CAD build for the part. Positions are in the model's coordinates, mm. A direction names the side the tool comes from. Coordinates: 2 decimals unless noted, no trailing zeros. Write each loop counter-clockwise with the first axis right and the second up, starting at its lowest first coordinate (ties: lowest second). Pieces come first, ordered by that corner, then holes. Notation, with made-up numbers: (42.5, 18.25) -> (96.5, 18.25) arc R10 cw to (96.5, 37.25) -> close; hole circle Ø6 at (21, 65.25). An arc over 180 degrees is marked (long way). Answer as CSV lines item,"result".
```python
from build123d import *

# Parameters (mm, degrees)
SKETCH_1_R          = 30
EXTRUDE_1_DEPTH     = 35
SKETCH_2_R          = 1.65
CUT_EXTRUDE_1_DEPTH = 56
SKETCH_4_R          = 20
CUT_EXTRUDE_3_DEPTH = 10
SKETCH_5_R          = 4
CUT_EXTRUDE_4_DEPTH = 50.244289009
SKETCH_6_R          = 2.15
SKETCH_6_R_2        = 1.55
CUT_EXTRUDE_5_DEPTH = 50.244289009


with BuildPart() as part:
    # 草图1 → 凸台-拉伸1 (new body)
    with BuildSketch(Plane(origin=(0, 0, 0), x_dir=(1, 0, 0), z_dir=(0, 1, 0))):
        with Locations(Location((0, 0, 0), (0, 0, 270))):
            Circle(SKETCH_1_R)
    extrude(amount=EXTRUDE_1_DEPTH)

    # 草图2 → 切除-拉伸1 (cut, through all)
    with BuildSketch(Plane.XZ):
        with Locations(Location((-26.25, 0, 0), (0, 0, 270))):
            Circle(SKETCH_2_R)
        with Locations(Location((-20.108666632, 16.873174754, 0), (0, 0, 270))):
            Circle(SKETCH_2_R)
        with Locations(Location((-4.558264664, 25.851203517, 0), (0, 0, 270))):
            Circle(SKETCH_2_R)
        with Locations(Location((13.125, 22.733166849, 0), (0, 0, 270))):
            Circle(SKETCH_2_R)
        with Locations(Location((24.666931296, 8.978028762, 0), (0, 0, 270))):
            Circle(SKETCH_2_R)
        with Locations(Location((24.666931296, -8.978028762, 0), (0, 0, 270))):
            Circle(SKETCH_2_R)
        with Locations(Location((13.125, -22.733166849, 0), (0, 0, 270))):
            Circle(SKETCH_2_R)
        with Locations(Location((-4.558264664, -25.851203517, 0), (0, 0, 270))):
            Circle(SKETCH_2_R)
        with Locations(Location((-20.108666632, -16.873174754, 0), (0, 0, 270))):
            Circle(SKETCH_2_R)
    extrude(amount=-CUT_EXTRUDE_1_DEPTH, mode=Mode.SUBTRACT)

    # 草图4 → 切除-拉伸3 (cut)
    with BuildSketch(Plane.XZ):
        with Locations(Location((0, 0, 0), (0, 0, 270))):
            Circle(SKETCH_4_R)
    extrude(amount=-CUT_EXTRUDE_3_DEPTH, mode=Mode.SUBTRACT)

    # 草图5 → 切除-拉伸4 (cut, through all)
    with BuildSketch(Plane.XZ.offset(-10)):
        with Locations(Location((0, 0, 0), (0, 0, 270))):
            Circle(SKETCH_5_R)
    extrude(amount=-CUT_EXTRUDE_4_DEPTH, mode=Mode.SUBTRACT)

    # 草图6 → 切除-拉伸5 (cut, through all)
    with BuildSketch(Plane.XZ.offset(-10)):
        with Locations(Location((0, 12, 0), (0, 0, 270))):
            Circle(SKETCH_6_R)
        with Locations(Location((12, 0, 0), (0, 0, 270))):
            Circle(SKETCH_6_R)
        with Locations(Location((0, -12, 0), (0, 0, 270))):
            Circle(SKETCH_6_R)
        with Locations(Location((-12, 0, 0), (0, 0, 270))):
            Circle(SKETCH_6_R)
        with Locations(Location((-5.656854249, -5.656854249, 0), (0, 0, 270))):
            Circle(SKETCH_6_R_2)
        with Locations(Location((-5.656854249, 5.656854249, 0), (0, 0, 270))):
            Circle(SKETCH_6_R_2)
        with Locations(Location((5.656854249, 5.656854249, 0), (0, 0, 270))):
            Circle(SKETCH_6_R_2)
        with Locations(Location((5.656854249, -5.656854249, 0), (0, 0, 270))):
            Circle(SKETCH_6_R_2)
    extrude(amount=-CUT_EXTRUDE_5_DEPTH, mode=Mode.SUBTRACT)


solid = part.part
```
Item 1: Flat gauge pins, fed straight in: pin 1 (2 mm diameter, centred on x = 24.67, z = 8.98, fed in from +Y); pin 2 (8 mm diameter, centred on y = 30, z = 18.5, fed in from -X); pin 3 (3.5 mm diameter, centred on x = -5.66, z = -5.66, fed in from -Y); pin 4 (10 mm diameter, centred on y = 6, z = -10, fed in from -X). Where does each tip first touch, or does it go through?
Answer below:
pin 1,"passes through"
pin 2,"stops at x = -26.26"
pin 3,"stops at y = 10"
pin 4,"stops at x = -29.58"
Item 2: Saw through at C-C on y = 7. State how many separate pieces and enclosed holes the cut face has, and give its area (3 significant figures).
Answer below:
separate pieces,"1"
enclosed holes,"10"
area,"1,490 mm2"
Item 3: Two-plate mould, pull along Z, no slides. Class faces 3 (the cylindrical face through (-24.614, 17.255, 0.215)), 4 (the cylindrical face through (0.65, 22.32, 9.95)), 5 (the flat face through (-6, 0, 20)): pulls with the +Z half, pulls with the -Z half, needs draft (parallel to the pull), parting line crosses it, or undercut.
Answer below:
face 3,"undercut"
face 4,"undercut"
face 5,"needs draft"
Item 4: Saw through at D-D on x = -12. Give the cut face in (y, z), and give its area (3 significant figures).
Answer below:
outline,"(0, -27.5) -> (35, -27.5) -> (35, -2.15) -> (10, -2.15) -> (10, -16) -> (0, -16) -> close; (0, 16) -> (10, 16) -> (10, 2.15) -> (35, 2.15) -> (35, 27.5) -> (0, 27.5) -> close"
area,"1,500 mm2"
Item 5: Saw through at B-B on x = 0. Give the cut face in (y, z).
Answer below:
outline,"(0, -30) -> (35, -30) -> (35, -14.15) -> (10, -14.15) -> (10, -20) -> (0, -20) -> close; (0, 20) -> (10, 20) -> (10, 14.15) -> (35, 14.15) -> (35, 30) -> (0, 30) -> close; (10, -9.85) -> (35, -9.85) -> (35, -4) -> (10, -4) -> close; (10, 4) -> (35, 4) -> (35, 9.85) -> (10, 9.85) -> close"
Item 6: 3-axis set-ups, long thin cutter, end or side, ignore diameter. For faces 1 (the cylindrical face through (-19.524, 4.93, 4.336)), 2 (the cylindrical face through (10.09, 22.32, -0.99)): which of +Z, -Z, +X, -X, +Y, -Y reach the whole face in a straight line?
Answer below:
face 1,"-Y"
face 2,"+Y, -Y"
Item 7: Saw through at A-A on z = 0. Give the cut face in (x, y).
Answer below:
outline,"(-30, 0) -> (-27.9, 0) -> (-27.9, 35) -> (-30, 35) -> close; (-24.6, 0) -> (-20, 0) -> (-20, 10) -> (-14.15, 10) -> (-14.15, 35) -> (-24.6, 35) -> close; (-9.85, 10) -> (-4, 10) -> (-4, 35) -> (-9.85, 35) -> close; (4, 10) -> (9.85, 10) -> (9.85, 35) -> (4, 35) -> close; (14.15, 10) -> (20, 10) -> (20, 0) -> (30, 0) -> (30, 35) -> (14.15, 35) -> close"
Item 8: Wall check: line 1 (X direction, y = 5, z = 0); line 2 (X direction, y = 28, z = 0); line 3 (X direction, y = 22, z = 12). Give the ranges that are in metal, low to high. Write a range as from..to.
Answer below:
line 1,"x = -30..-27.9, -24.6..-20, 20..30"
line 2,"x = -30..-27.9, -24.6..-14.15, -9.85..-4, 4..9.85, 14.15..30"
line 3,"x = -27.5..-2.15, 2.15..27.5"
